Read the model definition and answer for the solid it produces. Units are mm, in the model's axes. Face numbers are marked on the shaded views. A direction names the side the tool comes from. Coordinates: 2 decimals unless noted, no trailing zeros. Write each loop counter-clockwise with the first axis right and the second up, starting at its lowest first coordinate (ties: lowest second). Pieces come first, ordered by that corner, then holes.
Item 1: Section A-A (z = -4.5) is taken. Give the vertices of the cut face in (x, y).
Item 2: Section D-D (x = 4.5) is taken. Give the vertices of the cut face in (y, z), then the cut area to 4 significant figures.
Item 3: Section C-C (z = -2.5) is taken. Give the vertices of the cut face in (x, y).
Item 4: Straight lines are drawn through the part: probe 1 along Z at (x, y) = (13.1, 5.2); probe 2 along X at (y, z) = (9.75, -0.5); probe 3 along Y at (x, z) = (0.25, -3). For each, find the intervals that lie inside material, in ascending order.
Item 5: Each of these flat-tipped pins is pushed along its axis until it touches: P1, Ø7.5, axis at x = -0.5, z = -3.5, coming from the +Y side; P2, Ø2, axis at y = 5.2, z = 4.5, coming from the +X side; P3, Ø1.5, axis at y = 8, z = 3, coming from the -X side; P4, Ø1.1, axis at y = 5.2, z = -4.5, coming from the +X side. Where does it stop, or does it pass through?
Item 6: Section B-B (y = 5.2) is taken. Give the vertices of the cut face in (x, z).
Item 7: A tool of negligible diameter and unlimited length cuts with its end or side. For the marked faces 1 and 2, from which of +Z, -Z, +X, -X, +Y, -Y can it reach the whole face along a straight path? Write none if from no direction.
from build123d import *

# Parameters (mm, degrees)
SKETCH1_W                    = 25
SKETCH1_H                    = 15
BASE_FLANGE1_DEPTH           = 1.27
EDGE_FLANGE1_STRIP_W         = 6.5532
EDGE_FLANGE1_STRIP_H         = 1.27
EDGE_FLANGE1_STRIP_CUT_DEPTH = 15
EDGE_FLANGE1_DEPTH           = 15
M1_6_CLEARANCE_HOLE1_D       = 1.8


# Sheet-metal steps are written as plain solids
with BuildPart() as part:
    # Sketch1 → Base-Flange1 (new body)
    with BuildSketch(Plane(origin=(0, 0, 0), x_dir=(1, 0, 0), z_dir=(0, 1, 0))):
        Rectangle(SKETCH1_W, SKETCH1_H)
    extrude(amount=-BASE_FLANGE1_DEPTH)

    # Edge-Flange1 strip (across the edge) → Edge-Flange1 strip cut (cut)
    with BuildSketch(Plane(origin=(12.5, 0, 7.5), x_dir=(-1, 0, 0), z_dir=(0, 0, -1))):
        with Locations((-2.54, -0.635)):
            Rectangle(EDGE_FLANGE1_STRIP_W, EDGE_FLANGE1_STRIP_H)
    extrude(amount=EDGE_FLANGE1_STRIP_CUT_DEPTH, mode=Mode.SUBTRACT)

    # Edge-Flange1 section (across the edge) → Edge-Flange1 (add)
    with BuildSketch(Plane(origin=(12.5, 0, 7.5), x_dir=(-1, 0, 0), z_dir=(0, 0, -1))):
        with BuildLine():
            Line((-1.27, 0.7366), (-1.27, 10.2))
            Line((-1.27, 10.2), (0, 10.2))
            Line((0, 10.2), (0, 0.7366))
            ThreePointArc((0, 0.7366), (0.215745145, 0.215745145), (0.7366, 0))
            Line((0.7366, 0), (0.7366, -1.27))
            ThreePointArc((0.7366, -1.27), (-0.682280467, -0.682280467), (-1.27, 0.7366))
        make_face()
    extrude(amount=EDGE_FLANGE1_DEPTH)

    # M1.6 Clearance Hole1 (through all)
    with Locations(Plane(origin=(13.77, 5.2, 4.5), x_dir=(0, 1, 0), z_dir=(1, 0, 0))):
        with Locations((0, 0), (0, -9)):
            Hole(M1_6_CLEARANCE_HOLE1_D / 2)


solid = part.part
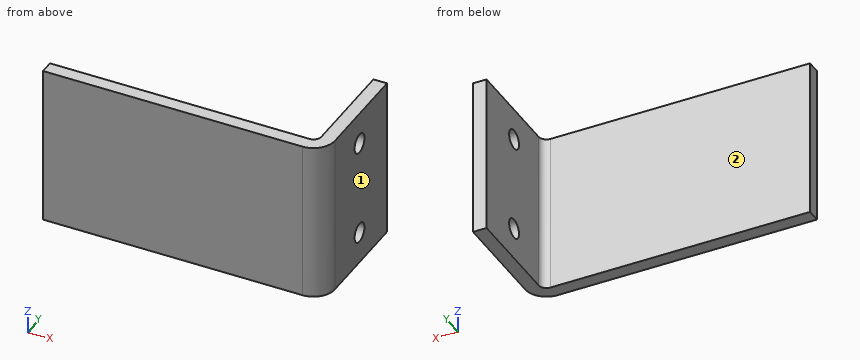
Established:
1. outline: (-12.5, -1.27) - (11.76, -1.27) arc R2.01 ccw to (13.77, 0.74) - (13.77, 4.3) - (12.5, 4.3) - (12.5, 0.74) arc R0.74 cw to (11.76, 0) - (-12.5, 0) - close; (12.5, 6.1) - (13.77, 6.1) - (13.77, 10.2) - (12.5, 10.2) - close
2. outline: (-1.27, -7.5) - (0, -7.5) - (0, 7.5) - (-1.27, 7.5) - close
2. area: 19.05 mm2
3. outline: (-12.5, -1.27) - (11.76, -1.27) arc R2.01 ccw to (13.77, 0.74) - (13.77, 10.2) - (12.5, 10.2) - (12.5, 0.74) arc R0.74 cw to (11.76, 0) - (-12.5, 0) - close
4. probe 1: z = -7.5 to -5.4, -3.6 to 3.6, 5.4 to 7.5
4. probe 2: x = 12.5 to 13.77
4. probe 3: y = -1.27 to 0
5. P1: stops at y = 0
5. P2: stops at x = 13.77
5. P3: stops at x = 12.5
5. P4: passes through
6. outline: (12.5, -7.5) - (13.77, -7.5) - (13.77, -5.4) - (12.5, -5.4) - close; (12.5, -3.6) - (13.77, -3.6) - (13.77, 3.6) - (12.5, 3.6) - close; (12.5, 5.4) - (13.77, 5.4) - (13.77, 7.5) - (12.5, 7.5) - close
7. face 1: +Z, -Z, +X, +Y, -Y
7. face 2: +Z, -Z, -X, +Y
